The model under review builds one solid part; all positions refer to its coordinate system, in mm. Face numbers are marked on the shaded views. A direction names the side the tool comes from. Give positions to 0.01 mm unless a question says otherwise; leave off trailing zeros. Loops run counter-clockwise (first coordinate to the right, second up) from the corner with the lowest first, then second, coordinate; pieces in that order, holes last. Notation, with made-up numbers: M -26.75,-13.75 L -2.75,-13.75 A28 cw -2.75,22.25 Z; hole C 1,59.5 d4. An arc over 180 degrees is marked long. Return JSON: item names as keys, results as strings. Group by question number.
```python
from build123d import *

# Parameters (mm, degrees)
ABC_DEPTH = 124.457734282


with BuildPart() as part:
    # Sketch15 → ABC (new body)
    with BuildSketch(Plane(origin=(0, 0, 0), x_dir=(0, -1, 0), z_dir=(-1, 0, 0))):
        with BuildLine():
            Line((-8, -9), (8, -9))
            ThreePointArc((8, -9), (8.707106781, -8.707106781), (9, -8))
            Line((9, -8), (9, 8))
            ThreePointArc((9, 8), (8.004363309, 8.999990481), (7.000038077, 8.008726535))
            Line((7.000038077, 8.008726535), (6.965131935, 4.008878843))
            Line((6.965131935, 4.008878843), (5.965170012, 4.017605379))
            Line((5.965170012, 4.017605379), (6.000076154, 8.017453071))
            ThreePointArc((6.000076154, 8.017453071), (8.008726619, 9.999980961), (10, 8))
            Line((10, 8), (10, -8))
            ThreePointArc((10, -8), (9.414213562, -9.414213562), (8, -10))
            Line((8, -10), (-8, -10))
            ThreePointArc((-8, -10), (-9.414213562, -9.414213562), (-10, -8))
            Line((-10, -8), (-10, 8))
            ThreePointArc((-10, 8), (-8.008726619, 9.999980961), (-6.000076154, 8.017453071))
            Line((-6.000076154, 8.017453071), (-5.965170012, 4.017605379))
            Line((-5.965170012, 4.017605379), (-6.965131935, 4.008878843))
            Line((-6.965131935, 4.008878843), (-7.000038077, 8.008726535))
            ThreePointArc((-7.000038077, 8.008726535), (-8.004363309, 8.999990481), (-9, 8))
            Line((-9, 8), (-9, -8))
            ThreePointArc((-9, -8), (-8.707106781, -8.707106781), (-8, -9))
        make_face()
    extrude(amount=ABC_DEPTH)


solid = part.part
```
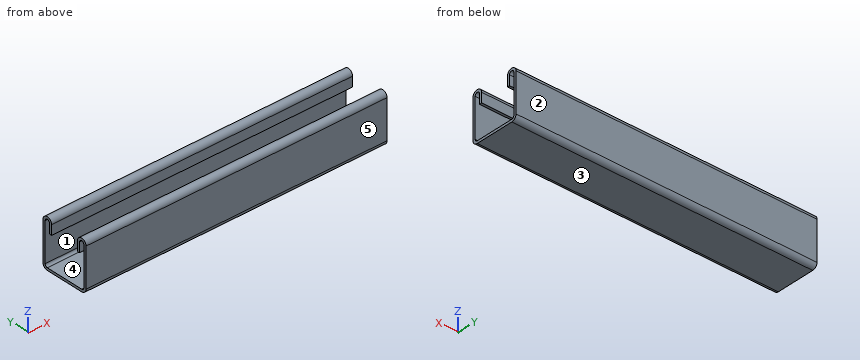
(1) Add section D-D (y = 4.5). Write out the cut boundary in (x, z), and give its area (3 significant figures).
(2) For pin 1 (1 mm diameter, centred on x = -84, y = -4, fed in from +Z); pin 2 (12 mm diameter, centred on x = -28, y = -1, fed in from +Z); pin 3 (3 mm diameter, centred on x = -29, y = 5, fed in from +Z), all flat-tipped, find the tip position at first contact; note any pin that passes through.
(3) For probe 1 along Y at (x, z) = (-97, 7); probe 2 along Y at (x, z) = (-21, -6); probe 3 along Y at (x, z) = (-6, 8.5), list the stretches that pass through material, from the lowest coordinate up.
(4) Add section B-B (x = -40.5). Write out the cut boundary in (y, z), and give its area (3 significant figures).
(5) Mouldability with a two-part tool opening along Z and no side actions: class the marked faces 3, 4 and 5 as released by +Z, released by -Z, zero draft, split by the parting line, or undercut.
(6) Add section C-C (z = 5.75). Write out the cut boundary in (x, y).
(7) For the marked faces 1 and 2, list the 3-axis set-ups (+Z, -Z, +X, -X, +Y, -Y) from which the entire face can be reached by the end or side of a thin tool; tool diameter is ignored.
(8) Add section A-A (z = -5). Write out the cut boundary in (x, y), and give its area (3 significant figures).
Verdict:
{
 "1": {"outline": "M -124.46,-10 L 0,-10 L 0,-9 L -124.46,-9 Z", "area": "124 mm²"},
 "2": {"pin 1": "stops at z = -9", "pin 2": "stops at z = 9.73", "pin 3": "stops at z = 9.32"},
 "3": {"probe 1": "y = -10 to -9, -6.99 to -5.99, 5.99 to 6.99, 9 to 10", "probe 2": "y = -10 to -9, 9 to 10", "probe 3": "y = -9.94 to -8.87, -7.13 to -6.06, 6.06 to 7.13, 8.87 to 9.94"},
 "4": {"outline": "M -10,-8 A2 ccw -8,-10 L 8,-10 A2 ccw 10,-8 L 10,8 A2 ccw 6,8.02 L 5.97,4.02 L 6.97,4.01 L 7,8.01 A1 cw 9,8 L 9,-8 A1 cw 8,-9 L -8,-9 A1 cw -9,-8 L -9,8 A1 cw -7,8.01 L -6.97,4.01 L -5.97,4.02 L -6,8.02 A2 ccw -10,8 Z", "area": "70.1 mm²"},
 "5": {"face 3": "released by -Z", "face 4": "undercut", "face 5": "zero draft"},
 "6": {"outline": "M -124.46,-10 L 0,-10 L 0,-9 L -124.46,-9 Z; M -124.46,-6.98 L 0,-6.98 L 0,-5.98 L -124.46,-5.98 Z; M -124.46,5.98 L 0,5.98 L 0,6.98 L -124.46,6.98 Z; M -124.46,9 L 0,9 L 0,10 L -124.46,10 Z"},
 "7": {"face 1": "+X, -X", "face 2": "+Z, -Z, +X, -X, +Y"},
 "8": {"outline": "M -124.46,-10 L 0,-10 L 0,-9 L -124.46,-9 Z; M -124.46,9 L 0,9 L 0,10 L -124.46,10 Z", "area": "249 mm²"}
}
